Geometry: final body of the model. Coordinates: model frame, mm. A direction names the side the tool comes from. Round coordinates to 2 decimals unless told otherwise and drop trailing zeros. Loops run counter-clockwise (first coordinate to the right, second up) from the corner with the lowest first, then second, coordinate; pieces in that order, holes last. Notation, with made-up numbers: M -8,47 L 28,47 A18 cw 28,64 Z; hole C -34,47 d8. An arc over 180 degrees is marked long. Write each question's results on one line, items separated by ' | '.
```python
from build123d import *

# Parameters (mm, degrees)
ESQUISSE1_W                  = 44.2
ESQUISSE1_H                  = 52.2
BOSS_EXTRU_1_DEPTH           = 52.2
ENL_V_MAT_EXTRU_2_DEPTH      = 74.209903702
ENL_V_MAT_EXTRU_2_DEPTH_BACK = 44.2
ENL_V_MAT_EXTRU_3_DEPTH      = 74.209903702
ENL_V_MAT_EXTRU_3_DEPTH_BACK = 44.2
ENL_V_MAT_EXTRU_4_DEPTH      = 78.059003368
ENL_V_MAT_EXTRU_4_DEPTH_BACK = 46
ENL_V_MAT_EXTRU_5_DEPTH      = 78.059003368
ENL_V_MAT_EXTRU_5_DEPTH_BACK = 46
ENL_V_MAT_EXTRU_7_DEPTH      = 45.550224466
ENL_V_MAT_EXTRU_7_DEPTH_BACK = 45.550224466
ENL_V_MAT_EXTRU_8_DEPTH      = 78.059003368
ENL_V_MAT_EXTRU_8_DEPTH_BACK = 46
ENL_V_MAT_EXTRU_9_DEPTH      = 75.993733072
ENL_V_MAT_EXTRU_9_DEPTH_BACK = 46
ESQUISSE13_R                 = 3
BOSS_EXTRU_2_DEPTH           = 21


with BuildPart() as part:
    # Esquisse1 → Boss.-Extru.1 (new body)
    with BuildSketch(Plane.XY):
        Rectangle(ESQUISSE1_W, ESQUISSE1_H)
    extrude(amount=BOSS_EXTRU_1_DEPTH)

    # Esquisse2 → Enlèv. mat.-Extru.2 (cut, two sides: drawn at the far end of the back side and taken through both)
    with BuildSketch(Plane(origin=(22.1, 0, 0), x_dir=(0, 0, -1), z_dir=(1, 0, 0)).offset(-ENL_V_MAT_EXTRU_2_DEPTH_BACK)):
        Polygon((-201.352290675, -19.9), (-52.2, -19.9), (-28.55, -19.9), (-28.55, -21.45), (-32.25, -21.45), (-32.25, -22.45), (-28.745559959, -26.1), (74.553898465, -133.690091099), (-39.180744024, -409.461834307), (-315.086933163, -295.671743208), align=None)
    extrude(amount=ENL_V_MAT_EXTRU_2_DEPTH + ENL_V_MAT_EXTRU_2_DEPTH_BACK, mode=Mode.SUBTRACT)

    # Esquisse3 → Enlèv. mat.-Extru.3 (cut, two sides: drawn at the far end of the back side and taken through both)
    with BuildSketch(Plane(origin=(22.1, 0, 0), x_dir=(0, 0, -1), z_dir=(1, 0, 0)).offset(-ENL_V_MAT_EXTRU_3_DEPTH_BACK)):
        Polygon((149.152290675, -19.9), (0, -19.9), (-23.65, -19.9), (-23.65, -21.45), (-19.95, -21.45), (-19.95, -22.45), (-23.454440041, -26.1), (-126.753898465, -133.690091099), (-13.019255976, -409.461834307), (262.886933163, -295.671743208), align=None)
    extrude(amount=ENL_V_MAT_EXTRU_3_DEPTH + ENL_V_MAT_EXTRU_3_DEPTH_BACK, mode=Mode.SUBTRACT)

    # Esquisse4 → Enlèv. mat.-Extru.4 (cut, two sides: drawn at the far end of the back side and taken through both)
    with BuildSketch(Plane(origin=(0, 26.1, 0), x_dir=(1, 0, 0), z_dir=(0, 1, 0)).offset(-ENL_V_MAT_EXTRU_4_DEPTH_BACK)):
        Polygon((-15.9, -191.333109619), (-15.9, -52.2), (-15.9, -28.55), (-17.45, -28.55), (-17.45, -32.25), (-18.45, -32.25), (-22.1, -28.745559959), (-122.462816227, 67.614843274), (-379.791464965, -38.281593439), (-273.228648738, -297.229546332), align=None)
    extrude(amount=ENL_V_MAT_EXTRU_4_DEPTH + ENL_V_MAT_EXTRU_4_DEPTH_BACK, mode=Mode.SUBTRACT)

    # Esquisse5 → Enlèv. mat.-Extru.5 (cut, two sides: drawn at the far end of the back side and taken through both)
    with BuildSketch(Plane(origin=(0, 26.1, 0), x_dir=(1, 0, 0), z_dir=(0, 1, 0)).offset(-ENL_V_MAT_EXTRU_5_DEPTH_BACK)):
        Polygon((-15.9, 139.133109619), (-15.9, 0), (-15.9, -23.65), (-17.45, -23.65), (-17.45, -19.95), (-18.45, -19.95), (-22.1, -23.454440041), (-122.462816228, -119.814843274), (-379.791464965, -13.918406561), (-273.228648738, 245.029546332), align=None)
    extrude(amount=ENL_V_MAT_EXTRU_5_DEPTH + ENL_V_MAT_EXTRU_5_DEPTH_BACK, mode=Mode.SUBTRACT)

    # Esquisse6 → Enlèv. mat.-Extru.7 (cut, two sides: drawn at the far end of the back side and taken through both)
    with BuildSketch(Plane.XY.offset(28.55).offset(-ENL_V_MAT_EXTRU_7_DEPTH_BACK)):
        Polygon((-161.22284167, -19.9), (-22.1, -19.9), (-15.9, -19.9), (-15.9, -26.093649616), (-15.9, -165.216491285), (-212.645110561, -361.97019968), (-357.967952231, -216.653708395), align=None)
    extrude(amount=ENL_V_MAT_EXTRU_7_DEPTH + ENL_V_MAT_EXTRU_7_DEPTH_BACK, mode=Mode.SUBTRACT)

    # Esquisse11 → Enlèv. mat.-Extru.8 (cut, two sides: drawn at the far end of the back side and taken through both)
    with BuildSketch(Plane(origin=(0, 26.1, 0), x_dir=(1, 0, 0), z_dir=(0, 1, 0)).offset(-ENL_V_MAT_EXTRU_8_DEPTH_BACK)):
        Polygon((164.227968273, -49.1), (22.1, -49.1), (-15.9, -49.1), (-158.027968273, -49.1), (-158.027968273, -333.355936546), (164.227968273, -333.355936546), align=None)
    extrude(amount=ENL_V_MAT_EXTRU_8_DEPTH + ENL_V_MAT_EXTRU_8_DEPTH_BACK, mode=Mode.SUBTRACT)

    # Esquisse12 → Enlèv. mat.-Extru.9 (cut, two sides: drawn at the far end of the back side and taken through both)
    with BuildSketch(Plane(origin=(0, 26.1, 0), x_dir=(1, 0, 0), z_dir=(0, 1, 0)).offset(-ENL_V_MAT_EXTRU_9_DEPTH_BACK)):
        Polygon((159.687460199, -3.1), (22.1, -3.1), (-15.9, -3.1), (-153.487460199, -3.1), (-153.487460199, 272.074920398), (159.687460199, 272.074920398), align=None)
    extrude(amount=ENL_V_MAT_EXTRU_9_DEPTH + ENL_V_MAT_EXTRU_9_DEPTH_BACK, mode=Mode.SUBTRACT)

    # Esquisse13 → Boss.-Extru.2 (add)
    with BuildSketch(Plane(origin=(22.1, 0, 0), x_dir=(0, 0, -1), z_dir=(1, 0, 0))):
        with Locations(Location((-27.1, 3.6, 0), (0, 0, 270))):
            Circle(ESQUISSE13_R)
    extrude(amount=BOSS_EXTRU_2_DEPTH)


solid = part.part
```
1. Pin query (flat end, axial travel): P1, Ø6, axis at x = -6.5, z = 41, coming from the -Y side; P2, Ø0.5, axis at x = -16.5, y = 9.5, coming from the +Z side; P3, Ø16.5, axis at y = 9, z = 39, coming from the -X side. Return the tip coordinate at first contact, or that it passes through.
Answer key:
P1: stops at y = -19.9 | P2: stops at z = 28.55 | P3: stops at x = -20.01
2. Section D-D (y = 20). Output: boundary loops of the cut face in (x, z), then the cut area to 3 significant figures.
Answer key:
outline: M -22.1,23.45 L -18.45,19.95 L -17.45,19.95 L -17.45,23.65 L -15.9,23.65 L -15.9,3.1 L 22.1,3.1 L 22.1,49.1 L -15.9,49.1 L -15.9,28.55 L -17.45,28.55 L -17.45,32.25 L -18.45,32.25 L -22.1,28.75 Z | area: 1,800 mm²
3. Section C-C (z = 27.1). Output: boundary loops of the cut face in (x, y), then the cut area to 3 significant figures.
Answer key:
outline: M -22.1,-19.9 L -15.9,-19.9 L -15.9,-26.1 L 22.1,-26.1 L 22.1,0.6 L 43.1,0.6 L 43.1,6.6 L 22.1,6.6 L 22.1,26.1 L -22.1,26.1 Z | area: 2,390 mm²
4. Section A-A (x = -12). Output: boundary loops of the cut face in (y, z).
Answer key:
outline: M -26.1,23.45 L -22.45,19.95 L -21.45,19.95 L -21.45,23.65 L -19.9,23.65 L -19.9,3.1 L 26.1,3.1 L 26.1,49.1 L -19.9,49.1 L -19.9,28.55 L -21.45,28.55 L -21.45,32.25 L -22.45,32.25 L -26.1,28.75 Z
5. Ray query, probe 1 along X at (y, z) = (16, 9.5); probe 2 along Y at (x, z) = (16.5, 17); probe 3 along X at (y, z) = (9.5, 28.5). Return the intervals inside material, ascending.
Answer key:
probe 1: x = -15.9 to 22.1 | probe 2: y = -19.9 to 26.1 | probe 3: x = -22.1 to 22.1
6. Draft query along Y for faces 5 (the face through (3, -21, 28.55)), 6 (the face through (-15.9, 3, 14)), 7 (the face through (2.83, -24.25, 30.52)), 8 (the face through (3, -21.45, 30)). Return one class per face: pulls with the +Y half, pulls with the -Y half, needs draft (parallel to the pull), parting line crosses it, or undercut.
Answer key:
face 5: undercut | face 6: needs draft | face 7: pulls with the -Y half | face 8: undercut
7. Section B-B (y = 3.6). Output: boundary loops of the cut face in (x, z), then the cut area to 3 significant figures.
Answer key:
outline: M -22.1,23.45 L -18.45,19.95 L -17.45,19.95 L -17.45,23.65 L -15.9,23.65 L -15.9,3.1 L 22.1,3.1 L 22.1,24.1 L 43.1,24.1 L 43.1,30.1 L 22.1,30.1 L 22.1,49.1 L -15.9,49.1 L -15.9,28.55 L -17.45,28.55 L -17.45,32.25 L -18.45,32.25 L -22.1,28.75 Z | area: 1,930 mm²
8. Access query for faces 1 (the face through (-19, -19.9, 26)), 2 (the face through (3, -21, 23.65)), 3 (the face through (-17.45, 3, 22)), 4 (the face through (-17, 3, 28.55)). Directions: +Z, -Z, +X, -X, +Y, -Y. A direction counts if a zero-diameter tool reaches every point of the face in a straight line with its end or side. Return the directions, or none.
Answer key:
face 1: +Z, -Z, -X, -Y | face 2: -Z, +X, -X | face 3: -Z, +Y, -Y | face 4: +Z, +Y, -Y
